Read the model definition and answer for the solid it produces. Units are mm, in the model's axes. A direction names the side the tool comes from. Coordinates: 2 decimals unless noted, no trailing zeros. Order: outer loops, then holes, each group sorted by start corner. A loop starts at its lowest first (then second) coordinate and runs counter-clockwise, first axis right, second up. Notation, with made-up numbers: M 67,-25 L 110,-25 A11 cw 110,-7 Z; hole C -34.5,67.25 d2. An arc over 180 degrees is marked long. Use a Markdown table: item, result. Add a question column.
1) Find section C-C on z = 6.35. Write down the section's boundary in (x, y) (3 decimals).
2) For faces 1 (the face through (0, 13, 25)), 2 (the face through (17, 22.225, 25)), determine the directions among +Z, -Z, +X, -X, +Y, -Y from which every point of the face is accessible in a straight line to the end or side of a thin tool.
3) The mould has two halves that part along Y. Classify faces 3 (the face through (2, 0, 25)), 4 (the face through (1.61, 13.74, 4.68)), 5 (the face through (25.4, 24, 25)): released by +Y, released by -Y, zero draft, split by the parting line, or undercut.
4) Each of these flat-tipped pins is pushed along its axis until it touches: pin 1 Ø3 at (y, z) = (18.5, 38) entering from +X (3 decimals); pin 2 Ø8 at (x, z) = (11, 24) entering from -Y (3 decimals). Where does it stop, or does it pass through?
5) Find section D-D on x = 23.5. Write down the section's boundary in (y, z) (3 decimals), plus the area to 3 significant figures.
6) Find the intervals of material crossed by probe 1 along Y at (x, z) = (1.25, 6.35); probe 2 along X at (y, z) = (23.6, 25.4); probe 3 along Y at (x, z) = (11.25, 28.5) (3 decimals), in increasing order. Write a range as [from, to].
7) Find section A-A on z = 25.4. Write down the section's boundary in (x, y) (3 decimals), plus the area to 3 significant figures.
8) Find section B-B on y = 23. Write down the section's boundary in (x, z).
from build123d import *

# Parameters (mm, degrees)
BOSS_EXTRUDE1_DEPTH    = 50.8
SKETCH6_R              = 3.1115
CUT_EXTRUDE1_DEPTH     = 4.175
F_10_CLEARANCE_HOLE2_D = 5.1054


with BuildPart() as part:
    # Sketch3 → Boss-Extrude1 (new body)
    with BuildSketch(Plane.XY):
        Polygon((0, 0), (0, 25.4), (25.4, 25.4), (25.4, 22.225), (3.175, 22.225), (3.175, 0), align=None)
    extrude(amount=BOSS_EXTRUDE1_DEPTH)

    # Sketch6 → Cut-Extrude1 (cut, through all)
    with BuildSketch(Plane(origin=(3.175, 0, 0), x_dir=(0, 0, -1), z_dir=(1, 0, 0))):
        with Locations((-44.45, 11.1125)):
            Circle(SKETCH6_R)
        with Locations((-6.35, 11.1125)):
            Circle(SKETCH6_R)
    extrude(amount=-CUT_EXTRUDE1_DEPTH, mode=Mode.SUBTRACT)

    # #10 Clearance Hole2 (through all)
    with Locations(Plane(origin=(0, 22.225, 0), x_dir=(-1, 0, 0), z_dir=(0, -1, 0))):
        with Locations((-14.2875, -25.4)):
            Hole(F_10_CLEARANCE_HOLE2_D / 2)


solid = part.part
Check result:
| question | item | result |
|---|---|---|
| 1 | outline | M 0,0 L 3.175,0 L 3.175,8.001 L 0,8.001 Z; M 0,14.224 L 3.175,14.224 L 3.175,22.225 L 25.4,22.225 L 25.4,25.4 L 0,25.4 Z |
| 2 | face 1 | +Z, -Z, -X, +Y, -Y |
| 2 | face 2 | +Z, -Z, +X, -Y |
| 3 | face 3 | released by -Y |
| 3 | face 4 | undercut |
| 3 | face 5 | zero draft |
| 4 | pin 1 | stops at x = 3.175 |
| 4 | pin 2 | stops at y = 22.225 |
| 5 | outline | M 22.225,0 L 25.4,0 L 25.4,50.8 L 22.225,50.8 Z |
| 5 | area | 161 mm2 |
| 6 | probe 1 | y = [0, 8], [14.22, 25.4] |
| 6 | probe 2 | x = [0, 11.73], [16.84, 25.4] |
| 6 | probe 3 | y = [22.225, 25.4] |
| 7 | outline | M 0,0 L 3.175,0 L 3.175,22.225 L 11.735,22.225 L 11.735,25.4 L 0,25.4 Z; M 16.84,22.225 L 25.4,22.225 L 25.4,25.4 L 16.84,25.4 Z |
| 7 | area | 135 mm2 |
| 8 | outline | M 0,0 L 25.4,0 L 25.4,50.8 L 0,50.8 Z; hole C 14.29,25.4 d5.11 |
